The model under review builds one solid part; all positions refer to its coordinate system, in mm. Face numbers are marked on the shaded views. A direction names the side the tool comes from. Give positions to 0.01 mm unless a question says otherwise; leave off trailing zeros. Loops run counter-clockwise (first coordinate to the right, second up) from the corner with the lowest first, then second, coordinate; pieces in that order, holes last. Notation, with made-up numbers: M 6,77 L 35,77 A31 cw 35,106 Z; hole C -31,50 d5. An arc over 180 degrees is marked long. Put each result on its own line as item: value. Start each with the question number.
```python
from build123d import *

# Parameters (mm, degrees)
BOSS_EXTRUDE1_DEPTH = 5.35


with BuildPart() as part:
    # Model → Boss-Extrude1 (new body)
    with BuildSketch(Plane.XY):
        with BuildLine():
            Line((10.342343988, 19.35), (10.483423975, 19.35))
            ThreePointArc((10.483423975, 19.35), (10.998948723, 19.20687469), (11.366904192, 18.818468468))
            ThreePointArc((11.366904192, 18.818468468), (12.610215159, 16.712376055), (14.040684229, 14.728640777))
            ThreePointArc((14.040684229, 14.728640777), (14.389100425, 14.449622517), (14.824210053, 14.35))
            Line((14.824210053, 14.35), (17.571488159, 14.35))
            ThreePointArc((17.571488159, 14.35), (17.946708443, 14.276935671), (18.26709829, 14.068419477))
            ThreePointArc((18.26709829, 14.068419477), (35, 7.295), (51.73290171, 14.068419477))
            ThreePointArc((51.73290171, 14.068419477), (52.053291557, 14.276935671), (52.428511841, 14.35))
            Line((52.428511841, 14.35), (55.175789947, 14.35))
            ThreePointArc((55.175789947, 14.35), (55.610899575, 14.449622517), (55.959315771, 14.728640777))
            ThreePointArc((55.959315771, 14.728640777), (57.389784841, 16.712376055), (58.633095808, 18.818468468))
            ThreePointArc((58.633095808, 18.818468468), (59.001051277, 19.20687469), (59.516576025, 19.35))
            Line((59.516576025, 19.35), (59.657656012, 19.35))
            ThreePointArc((59.657656012, 19.35), (60.201987066, 19.511129507), (60.570902531, 19.942592593))
            ThreePointArc((60.570902531, 19.942592593), (62.28136196, 25.047041201), (62.9833482, 30.384482759))
            ThreePointArc((62.9833482, 30.384482759), (63.287945159, 31.069194952), (63.982753492, 31.35))
            Line((63.982753492, 31.35), (70, 31.35))
            Line((70, 31.35), (70, 18.35))
            Line((70, 18.35), (65, 18.35))
            Line((65, 18.35), (65, 13))
            Line((65, 13), (70, 13))
            Line((70, 13), (70, 0))
            Line((70, 0), (64, 0))
            Line((64, 0), (64, 5.35))
            Line((64, 5.35), (6, 5.35))
            Line((6, 5.35), (6, 0))
            Line((6, 0), (0, 0))
            Line((0, 0), (0, 13))
            Line((0, 13), (5, 13))
            Line((5, 13), (5, 18.35))
            Line((5, 18.35), (0, 18.35))
            Line((0, 18.35), (0, 31.35))
            Line((0, 31.35), (6.017246508, 31.35))
            ThreePointArc((6.017246508, 31.35), (6.712054841, 31.069194952), (7.0166518, 30.384482759))
            ThreePointArc((7.0166518, 30.384482759), (7.71863804, 25.047041201), (9.429097469, 19.942592593))
            ThreePointArc((9.429097469, 19.942592593), (9.798012934, 19.511129507), (10.342343988, 19.35))
        make_face()
    extrude(amount=BOSS_EXTRUDE1_DEPTH)


solid = part.part
```
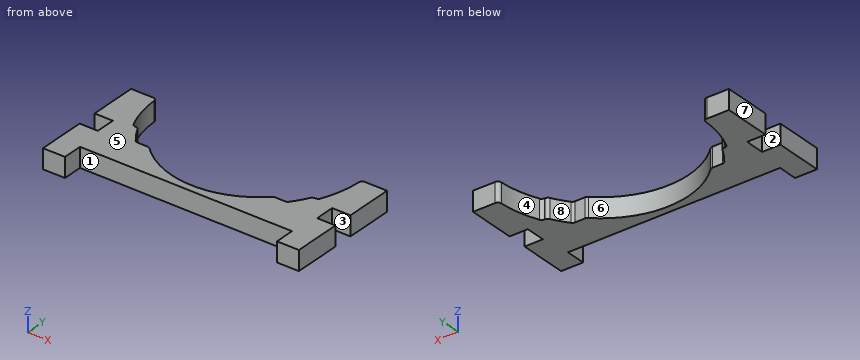
Item 1: Consider section C-C, the plane x = 58. Write out the cut boundary in (y, z), plus the area to 3 significant figures.
Item 2: To check wall thickness, follow L1, parallel to X at y = 5, z = 0.95; L2, parallel to X at y = 20.5, z = 0.95; L3, parallel to Y at x = 53.5, z = 3.85. State the ranges of each line that lie inside material, in increasing order. Write a range as [from, to].
Item 3: Clearance check with flat-ended pins moving along their axes: pin 1 Ø1.4 at (x, z) = (15.5, 4) entering from +Y; pin 2 Ø1.6 at (y, z) = (16.5, 3.5) entering from +X; pin 3 Ø1.6 at (x, z) = (25.5, 2.5) entering from -Y. State where each tip first meets the part, or that it passes through.
Item 4: Consider section B-B, the plane y = 11.5. Write out the cut boundary in (x, z), plus the area to 3 significant figures.
Item 5: Draft analysis for pull direction X (two halves, no side actions). For the marked faces 5, 6, 7 and 8, state which applies: +X half, -X half, draft (parallel to the pull), parting line (faces both ways), or undercut.
Item 6: Tool access review of the marked faces 1, 2, 3 and 4: name each direction out of +Z, -Z, +X, -X, +Y, -Y from which nothing blocks a thin tool from reaching the whole face with its end or side.
Item 7: Consider section D-D, the plane x = 38.5. Write out the cut boundary in (y, z).
Item 8: Consider section A-A, the plane y = 27.5. Write out the cut boundary in (x, z), plus the area to 3 significant figures.
Report:
1. outline: M 5.35,0 L 17.69,0 L 17.69,5.35 L 5.35,5.35 Z
1. area: 66.0 mm²
2. L1: [0, 6], [64, 70]
2. L2: [0, 9.19], [60.81, 70]
2. L3: [5.35, 14.35]
3. pin 1: y = 14.35
3. pin 2: x = 65
3. pin 3: y = 5.35
4. outline: M 0,0 L 21.41,0 L 21.41,5.35 L 0,5.35 Z; M 48.59,0 L 70,0 L 70,5.35 L 48.59,5.35 Z
4. area: 229 mm²
5. face 5: draft
5. face 6: undercut
5. face 7: -X half
5. face 8: undercut
6. face 1: +Z, -Z, -Y
6. face 2: +Z, -Z, -X
6. face 3: +Z, -Z, +X
6. face 4: +Z, -Z, +Y
7. outline: M 5.35,0 L 7.55,0 L 7.55,5.35 L 5.35,5.35 Z
8. outline: M 0,0 L 7.27,0 L 7.27,5.35 L 0,5.35 Z; M 62.73,0 L 70,0 L 70,5.35 L 62.73,5.35 Z
8. area: 77.7 mm²
